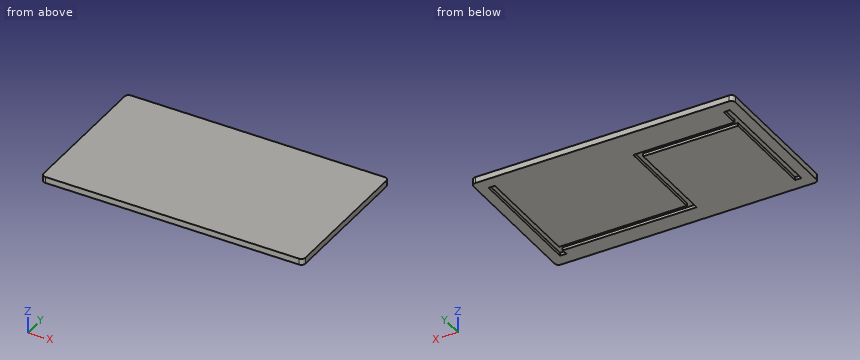
from build123d import *

# Parameters (mm, degrees)
F0_W     = 812.8
F0_H     = 457.2
F1_DEPTH = 19.05
F2_R     = 12.7
F3_W     = 19.446875
F3_H     = 18.653125
F3_H_2   = 266.7
F4_DEPTH = 9.525
F5_W     = 19.446875
F5_H     = 381
F6_DEPTH = 9.525
F7_W     = 313.928125
F7_H     = 19.446875
F7_W_2   = 415.925
F8_DEPTH = 9.525


with BuildPart() as f1:
    # F0 (on Top) → F1 (new body)
    with BuildSketch(Plane.XY):
        Rectangle(F0_W, F0_H)
    extrude(amount=F1_DEPTH)

    # F2
    f2_edges = [f1.edges().sort_by_distance(p)[0] for p in [
        (-406.4, -228.6, 9.525),
        (406.4, -228.6, 9.525),
        (406.4, 228.6, 9.525),
        (-406.4, 228.6, 9.525),
    ]]
    fillet(f2_edges, radius=F2_R)

    # F3 (on face) → F4 (cut)
    with BuildSketch(Plane(origin=(0, 0, 0), x_dir=(1, 0, 0), z_dir=(0, 0, -1))):
        with Locations((-50.998437, 142.676562)):
            Rectangle(F3_W, F3_H)
        with Locations((-50.998437, 0)):
            Rectangle(F3_W, F3_H_2)
    extrude(amount=-F4_DEPTH, mode=Mode.SUBTRACT)

    # F5 (on face) → F6 (cut)
    with BuildSketch(Plane(origin=(0, 0, 0), x_dir=(1, 0, 0), z_dir=(0, 0, -1))):
        with Locations((364.926562, 0)):
            Rectangle(F5_W, F5_H)
        with Locations((-364.926562, 0)):
            Rectangle(F5_W, F5_H)
    extrude(amount=-F6_DEPTH, mode=Mode.SUBTRACT)

    # F7 (on face) → F8 (cut)
    with BuildSketch(Plane(origin=(0, 0, 0), x_dir=(1, 0, 0), z_dir=(0, 0, -1))):
        with Locations((-198.239062, -123.626562)):
            Rectangle(F7_W, F7_H)
        with Locations((147.240625, 161.726562)):
            Rectangle(F7_W_2, F7_H)
    extrude(amount=-F8_DEPTH, mode=Mode.SUBTRACT)


solid = f1.part
Verification items for the finished model (mm, model axes). Round coordinates to 2 decimals unless told otherwise and drop trailing zeros. Loops run counter-clockwise (first coordinate to the right, second up) from the corner with the lowest first, then second, coordinate; pieces in that order, holes last. Notation, with made-up numbers: (-14.75, 2) - (39.25, 2) arc R18 ccw to (39.25, 14) - close; hole circle Ø6 at (23.5, 19). An arc over 180 degrees is marked (long way). Answer in a Markdown table with one row per item. Add a question column.
Q1. Material ranges on line 1 (X direction, y = 146.5, z = 2); line 2 (X direction, y = 116.5, z = 6.5) (3 decimals); line 3 (X direction, y = -134, z = 3.5) (3 decimals), recorded low to high.
Q2. Section check A-A on z = 4.5. Enter the section's corners in (x, y) (3 decimals), plus the area to 3 significant figures.
Q3. Section check B-B on x = -174.5. Enter the section's corners in (y, z) (3 decimals), plus the area to 3 significant figures.
Q4. Gauge pin test, flat end, axial feed: pin 1 (1.5 mm diameter, centred on x = 242.5, y = 13.5, fed in from -Z). Record the tip position at first contact, or that the pin passes through.
Q5. Section check C-C on y = -85. Enter the section's corners in (x, z) (3 decimals), plus the area to 3 significant figures.
Found:
| question | item | result |
|---|---|---|
| 1 | line 1 | x = -406.4 to -374.65, -355.2 to 355.2, 374.65 to 406.4 |
| 1 | line 2 | x = -406.4 to -374.65, -41.275 to 355.203, 374.65 to 406.4 |
| 1 | line 3 | x = -406.4 to -374.65, -355.203 to -60.722, -41.275 to 355.203, 374.65 to 406.4 |
| 2 | outline | (-406.4, -215.9) arc R12.7 ccw to (-393.7, -228.6) - (393.7, -228.6) arc R12.7 ccw to (406.4, -215.9) - (406.4, 215.9) arc R12.7 ccw to (393.7, 228.6) - (-393.7, 228.6) arc R12.7 ccw to (-406.4, 215.9) - close; hole (-374.65, -190.5) - (-355.203, -190.5) - (-355.203, 113.903) - (-60.722, 113.903) - (-60.722, -171.45) - (355.203, -171.45) - (355.203, -190.5) - (374.65, -190.5) - (374.65, 190.5) - (355.203, 190.5) - (355.203, -152.003) - (-41.275, -152.003) - (-41.275, 133.35) - (-355.203, 133.35) - (-355.203, 190.5) - (-374.65, 190.5) - close |
| 2 | area | 337,000 mm² |
| 3 | outline | (-228.6, 0) - (113.903, 0) - (113.903, 9.525) - (133.35, 9.525) - (133.35, 0) - (228.6, 0) - (228.6, 19.05) - (-228.6, 19.05) - close |
| 3 | area | 8,520 mm² |
| 4 | pin 1 | stops at z = 0 |
| 5 | outline | (-406.4, 0) - (-374.65, 0) - (-374.65, 9.525) - (-355.203, 9.525) - (-355.203, 0) - (-60.722, 0) - (-60.722, 9.525) - (-41.275, 9.525) - (-41.275, 0) - (355.203, 0) - (355.203, 9.525) - (374.65, 9.525) - (374.65, 0) - (406.4, 0) - (406.4, 19.05) - (-406.4, 19.05) - close |
| 5 | area | 14,900 mm² |
